Autodesk Fusion 360 part; units mm, degrees
box "BoxPrimitive1" add length 68.5 width 145 height 14 placed x (0, 0, -1) y (-1, 0, 0) z (0, 1, 0) at (145, 0, 0)
sketch "USB1" plane through (0, 0, 0) normal (-1, 0, 0) x (0, -1, 0)
  line L0 (-14, -68.5) -> (0, -68.5)
  line L1 (0, -68.5) -> (0, 0)
  line L2 (0, 0) -> (-14, 0)
  line L3 (-14, 0) -> (-14, -68.5)
  line L4 (-4.75, -60.5) -> (-9.75, -60.5)
  line L5 (-9.75, -60.5) -> (-9.75, -47.5)
  line L6 (-9.75, -47.5) -> (-4.75, -47.5)
  line L7 (-4.75, -47.5) -> (-4.75, -60.5)
  dimension "d14" = 5
  dimension "d15" = 13
  dimension "d16" = 8
  dimension "d17" = 4.25
extrude "Extrude3" cut sketch "USB1" against normal blind 20 contours L4 L5 L6 L7
sketch "USB4" plane through (0, 0, 0) normal (-1, 0, 0) x (0, -1, 0)
  line L0 (-14, -68.5) -> (0, -68.5)
  line L1 (0, -68.5) -> (0, 0)
  line L2 (-14, 0) -> (-14, -68.5)
  line L3 (-9.75, -21) -> (-4.75, -21)
  line L4 (-4.75, -21) -> (-4.75, -8)
  line L5 (-4.75, -8) -> (-9.75, -8)
  line L6 (-9.75, -8) -> (-9.75, -21)
  line L7 (0, 0) -> (-14, 0)
  dimension "d21" = 13
  dimension "d22" = 4.25
  dimension "d23" = 5
  dimension "d53" = 8
extrude "Extrude2" cut sketch "USB4" against normal blind 20 contours L3 L4 L5 L6
sketch "Sketch9" plane through (0, 0, 0) normal (-1, 0, 0) x (0, -1, 0)
  line L0 (-5, -44.5) -> (-8, -44.5)
  line L1 (-8, -44.5) -> (-8, -36.5)
  line L2 (-8, -36.5) -> (-5, -36.5)
  line L3 (-5, -36.5) -> (-5, -44.5)
  line L4 (0, -68.5) -> (0, 0)
  line L5 (-9.75, -47.5) -> (-4.75, -47.5)
  dimension "d34" = 8
  dimension "d35" = 3
  dimension "d36" = 5
  dimension "d37" = 3
extrude "Extrude4" cut sketch "Sketch9" against normal blind 10
sketch "Sketch10" plane through (0, 0, 0) normal (-1, 0, 0) x (0, -1, 0)
  line L0 (-4, -34.5) -> (-7, -34.5)
  line L1 (-7, -34.5) -> (-7, -25.5)
  line L2 (-7, -25.5) -> (-4, -25.5)
  line L3 (-4, -25.5) -> (-4, -34.5)
  line L4 (0, -68.5) -> (0, 0)
  line L5 (-9.75, -21) -> (-4.75, -21)
  dimension "d40" = 3
  dimension "d41" = 9
  dimension "d42" = 4
  dimension "d43" = 4.5
extrude "Extrude5" cut sketch "Sketch10" against normal blind 10
sketch "Sketch12" plane through (0, 0, 0) normal (0, 0, 1) x (-1, 0, 0)
  line L0 (0, 0) -> (-145, 0)
  line L1 (-145, 0) -> (-145, -14)
  line L2 (-145, -14) -> (0, -14)
  line L3 (0, 0) -> (0, -13.5)
sketch "Sketch15" plane through (0, 0, -68.5) normal (0, 0, -1) x (1, 0, 0)
  line L0 (145, -14) -> (145, 0)
  line L1 (145, 0) -> (0, 0)
  line L2 (0, 0) -> (0, -14)
  line L3 (0, -14) -> (145, -14)
  line L4 (15, -9.5) -> (25, -9.5)
  line L5 (25, -9.5) -> (25, -4.5)
  line L6 (25, -4.5) -> (15, -4.5)
  line L7 (15, -4.5) -> (15, -9.5)
The listing builds one solid part. Answer for the finished solid, in the listing's coordinates (mm). A direction names the side the tool comes from. Round coordinates to 2 decimals unless told otherwise and drop trailing zeros. Loops run counter-clockwise (first coordinate to the right, second up) from the corner with the lowest first, then second, coordinate; pieces in that order, holes last. Notation, with made-up numbers: M 46.5,-29 L 95.5,-29 A18 cw 95.5,-15 Z; hole C 56,35 d1. An arc over 180 degrees is marked long. Write each question's results on one line, items separated by ' | '. Start each with the question number.
1) Find section A-A on x = 14.5. Write down the section's boundary in (y, z).
2) Which of the six approach directions +Z, -Z, +X, -X, +Y, -Y give full straight-line access (tool end or side, diameter ignored) to faces 4 (the flat face through (20, 7, -14)), 5 (the flat face through (74, 7, 0))?
3) This flat-tipped pin is pushed along its axis until it touches: pin 1 (4 mm diameter, centred on y = 7, z = -14, fed in from -X). Where does it stop, or does it pass through?
4) Find section B-B on z = -11.5. Write down the section's boundary in (x, y), plus the area to 3 significant figures.
5) Determine the mould class of faces 1 (the flat face through (20, 7, -54)), 2 (the flat face through (71, 0, -34)), 3 (the flat face through (74, 7, -68.5)) for opening direction Y: pulls with the +Y half, pulls with the -Y half, needs draft (parallel to the pull), parting line crosses it, or undercut.
6) Straight lines are drawn through the part: probe 1 along Z at (x, y) = (9, 5.5); probe 2 along Y at (x, z) = (10, -13); probe 3 along X at (y, z) = (5, -10). For each, find the intervals that lie inside material, in ascending order.
Final values:
1) outline: M 0,-68.5 L 14,-68.5 L 14,0 L 0,0 Z; hole M 4.75,-60.5 L 9.75,-60.5 L 9.75,-47.5 L 4.75,-47.5 Z; hole M 4.75,-21 L 9.75,-21 L 9.75,-8 L 4.75,-8 Z
2) face 4: -X | face 5: +Z, +X, -X, +Y, -Y
3) pin 1: x = 20
4) outline: M 0,0 L 145,0 L 145,14 L 0,14 L 0,9.75 L 20,9.75 L 20,4.75 L 0,4.75 Z | area: 1,930 mm²
5) face 1: undercut | face 2: pulls with the -Y half | face 3: needs draft
6) probe 1: -68.5 to -60.5, -47.5 to -44.5, -36.5 to -34.5, -25.5 to -21, -8 to 0 | probe 2: 0 to 4.75, 9.75 to 14 | probe 3: 20 to 145
